Build history of the part. All positions in model axes, mm. Face numbers are marked on the shaded views. A direction names the side the tool comes from. Coordinates: 2 decimals unless noted, no trailing zeros. Order: outer loops, then holes, each group sorted by start corner. A loop starts at its lowest first (then second) coordinate and runs counter-clockwise, first axis right, second up. Notation, with made-up numbers: (-8.5, 72) - (50.5, 72) arc R23 cw to (50.5, 104) - close; hole circle Ø2 at (72.25, 83.25). An arc over 180 degrees is marked (long way). One line per item, written item: value.
from build123d import *

# Parameters (mm, degrees)
SKETCH_1_R          = 1.65
EXTRUDE_1_DEPTH     = 30
SKETCH_2_W          = 14
SKETCH_2_H          = 22
CUT_EXTRUDE_1_DEPTH = 30
SKETCH_3_W          = 18
SKETCH_3_H          = 22
CUT_EXTRUDE_2_DEPTH = 30
FILLET_1_R          = 3
SKETCH_4_R          = 1.65
CUT_EXTRUDE_3_DEPTH = 30
SKETCH_5_R          = 1.5
CUT_EXTRUDE_4_DEPTH = 45.418464629


with BuildPart() as part:
    # 草图1 → 凸台-拉伸1 (new body)
    with BuildSketch(Plane.XY):
        with BuildLine():
            Line((0, 0), (32, 0))
            Line((32, 0), (32, 6))
            ThreePointArc((32, 6), (30.048000097, 9.963545813), (25.716121836, 10.832355208))
            Line((25.716121836, 10.832355208), (0, 4))
            Line((0, 4), (0, 0))
        make_face()
        with Locations((27, 6)):
            Circle(SKETCH_1_R, mode=Mode.SUBTRACT)
    extrude(amount=EXTRUDE_1_DEPTH)

    # 草图2 → 切除-拉伸1 (cut)
    with BuildSketch(Plane.XZ):
        with Locations((25, 15)):
            Rectangle(SKETCH_2_W, SKETCH_2_H)
    extrude(amount=-CUT_EXTRUDE_1_DEPTH, mode=Mode.SUBTRACT)

    # 草图3 → 切除-拉伸2 (cut)
    with BuildSketch(Plane(origin=(0, 4, 0), x_dir=(-1, 0, 0), z_dir=(0, -1, 0))):
        with Locations((-9, -15)):
            Rectangle(SKETCH_3_W, SKETCH_3_H)
    extrude(amount=-CUT_EXTRUDE_2_DEPTH, mode=Mode.SUBTRACT)

    # 圆角1
    fillet_1_edges = [part.edges().sort_by_distance(p)[0] for p in [
        (18, 2, 26),
        (18, 2, 4),
    ]]
    fillet(fillet_1_edges, radius=FILLET_1_R)

    # 草图4 → 切除-拉伸3 (cut)
    with BuildSketch(Plane(origin=(0, 4, 0), x_dir=(1, 0, 0), z_dir=(0, 1, 0))):
        with Locations(Location((4, -15, 0), (0, 0, 270))):
            Circle(SKETCH_4_R)
    extrude(amount=-CUT_EXTRUDE_3_DEPTH, mode=Mode.SUBTRACT)

    # 草图5 → 切除-拉伸4 (cut, through all)
    with BuildSketch(Plane(origin=(0, 4, 0), x_dir=(1, 0, 0), z_dir=(0, 1, 0))):
        with Locations(Location((11, -10, 0), (0, 0, 270))):
            Circle(SKETCH_5_R)
        with Locations(Location((11, -20, 0), (0, 0, 270))):
            Circle(SKETCH_5_R)
    extrude(amount=-CUT_EXTRUDE_4_DEPTH, mode=Mode.SUBTRACT)


solid = part.part
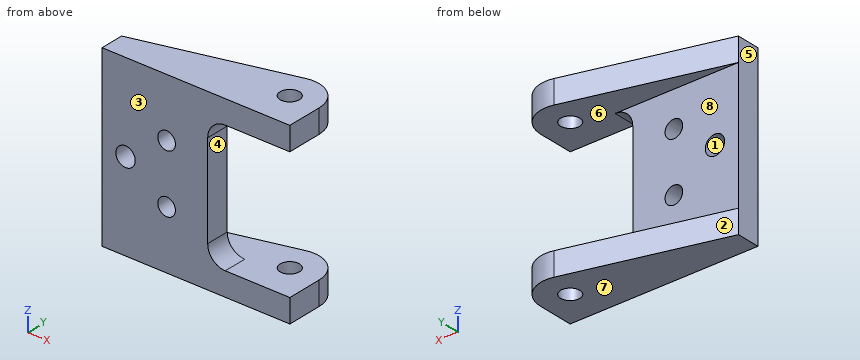
1. Band-saw the part on D-D, the plane z = 15. Give the cut face in (x, y).
Values found:
outline: (0, 0) - (2.35, 0) - (2.35, 4) - (0, 4) - close; (5.65, 0) - (18, 0) - (18, 4) - (5.65, 4) - close
2. Band-saw the part on A-A, the plane z = 20. Give the cut face in (x, y).
Values found:
outline: (0, 0) - (9.5, 0) - (9.5, 4) - (0, 4) - close; (12.5, 0) - (18, 0) - (18, 4) - (12.5, 4) - close
3. Band-saw the part on B-B, the plane y = 2.5. Give the cut face in (x, z).
Values found:
outline: (0, 0) - (32, 0) - (32, 4) - (21, 4) arc R3 cw to (18, 7) - (18, 23) arc R3 cw to (21, 26) - (32, 26) - (32, 30) - (0, 30) - close; hole circle Ø3.3 at (4, 15); hole circle Ø3 at (11, 10); hole circle Ø3 at (11, 20)
4. 3-axis set-ups, long thin cutter, end or side, ignore diameter. For the marked faces 4, 5, 6, 7 and 8: which of +Z, -Z, +X, -X, +Y, -Y reach the whole face in a straight line?
Values found:
face 4: +X, +Y, -Y
face 5: +Z, -Z, -X, +Y, -Y
face 6: +X, +Y
face 7: -Z, +X, -X, +Y, -Y
face 8: +X, -X, +Y
5. Band-saw the part on C-C, the plane x = 3. Give the cut face in (y, z), and give its area (3 significant figures).
Values found:
outline: (0, 0) - (4.8, 0) - (4.8, 4) - (4, 4) - (4, 13.69) - (0, 13.69) - close; (0, 16.31) - (4, 16.31) - (4, 26) - (4.8, 26) - (4.8, 30) - (0, 30) - close
area: 116 mm2
6. Flat gauge pins, fed straight in: P1, Ø2, axis at y = 2.5, z = 15.5, coming from the +X side; P2, Ø5, axis at x = 7, z = 26.5, coming from the +Y side; P3, Ø17, axis at x = 14.5, z = 17, coming from the +Y side. Where does each tip first touch, or does it go through?
Values found:
P1: stops at x = 18
P2: stops at y = 6.52
P3: stops at y = 4
7. Probe line 1 along X through (y, z) = (2.45, 10); line 2 along Z through (x, y) = (28.5, 10); line 3 along Y through (x, z) = (15.5, 23.25). List the from-to ranges inside material, lowest first.
Values found:
line 1: x = 0 to 9.5, 12.5 to 18
line 2: z = 0 to 4, 26 to 30
line 3: y = 0 to 4
8. Two-plate mould, pull along X, no slides. Class the marked faces 1, 2 and 3: pulls with the +X half, pulls with the -X half, needs draft (parallel to the pull), parting line crosses it, or undercut.
Values found:
face 1: undercut
face 2: pulls with the -X half
face 3: needs draft
